Read the model definition and answer for the solid it produces. Units are mm, in the model's axes. Face numbers are marked on the shaded views. A direction names the side the tool comes from. Give positions to 0.01 mm unless a question says otherwise; leave off trailing zeros. Write each loop counter-clockwise with the first axis right and the second up, starting at its lowest first coordinate (ties: lowest second). Pieces come first, ordered by that corner, then holes.
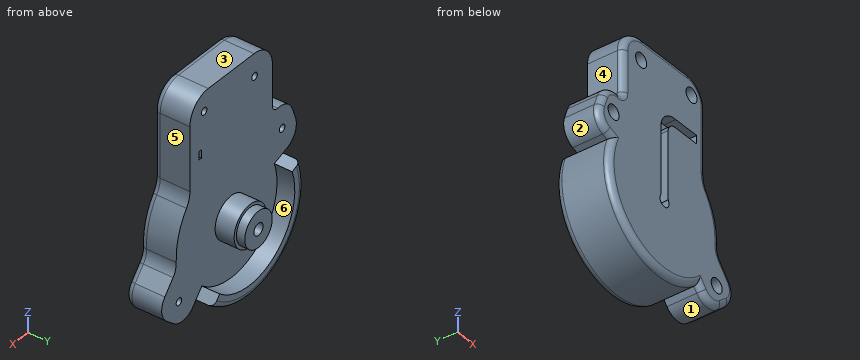
```python
from build123d import *

# Parameters (mm, degrees)
BOSS_EXTRUDE1_DEPTH = 30
SKETCH3_R           = 6
CUT_EXTRUDE2_DEPTH  = 10
CUT_EXTRUDE3_REACH  = 22
SKETCH4_R           = 3
SKETCH5_R           = 17.5
BOSS_EXTRUDE2_DEPTH = 16
SKETCH6_R           = 15
BOSS_EXTRUDE3_DEPTH = 7
BOSS_EXTRUDE4_DEPTH = 15
FILLET1_R           = 5
CUT_EXTRUDE4_REACH  = 55
SKETCH8_R           = 5
CUT_EXTRUDE5_REACH  = 32
SKETCH9_W           = 2.838035454
SKETCH9_H           = 7.000000767
CUT_EXTRUDE6_DEPTH  = 10


with BuildPart() as part:
    # Sketch1 → Boss-Extrude1 (new body)
    with BuildSketch(Plane(origin=(0, 0, 0), x_dir=(-1, 0, 0), z_dir=(0, -1, 0))):
        with BuildLine():
            Line((-155.978842812, -669.571630145), (-160.685424707, -671.259257732))
            ThreePointArc((-160.685424707, -671.259257732), (-169.1867086, -678.974834226), (-169.742287629, -690.441886175))
            Line((-169.742287629, -690.441886175), (-166.367032456, -699.855049964))
            ThreePointArc((-166.367032456, -699.855049964), (-160.015233889, -707.624119417), (-150.186716753, -709.649961495))
            ThreePointArc((-150.186716753, -709.649961495), (-146.216133795, -710.831997076), (-144.49986008, -714.602559592))
            Line((-144.49986008, -714.602559592), (-144.49986008, -749.320099104))
            ThreePointArc((-144.49986008, -749.320099104), (-138.641995704, -763.462234727), (-124.49986008, -769.320099104))
            Line((-124.49986008, -769.320099104), (-74.49986008, -769.320099104))
            ThreePointArc((-74.49986008, -769.320099104), (-60.357724456, -763.462234727), (-54.49986008, -749.320099104))
            Line((-54.49986008, -749.320099104), (-54.49986008, -695.956994369))
            ThreePointArc((-54.49986008, -695.956994369), (-53.539292845, -689.833270012), (-50.74986008, -684.297770553))
            ThreePointArc((-50.74986008, -684.297770553), (-41.916134266, -666.175796103), (-39.583621808, -646.150810326))
            ThreePointArc((-39.583621808, -646.150810326), (-38.838622962, -640.626520742), (-36.127881434, -635.755722136))
            Line((-36.127881434, -635.755722136), (-27.159022918, -624.993091916))
            ThreePointArc((-27.159022918, -624.993091916), (-23.743944015, -614.032289731), (-29.079576117, -603.867006728))
            Line((-29.079576117, -603.867006728), (-36.761788913, -597.465162731))
            ThreePointArc((-36.761788913, -597.465162731), (-47.722591099, -594.050083828), (-57.887874102, -599.38571593))
            Line((-57.887874102, -599.38571593), (-61.0887961, -603.226822328))
            ThreePointArc((-61.0887961, -603.226822328), (-133.880389498, -600.14714722), (-155.978842812, -669.571630145))
        make_face()
    extrude(amount=BOSS_EXTRUDE1_DEPTH)

    # Sketch3 → Cut-Extrude2 (cut)
    with BuildSketch(Plane.XZ.offset(30)):
        with Locations((42.52344851, 612.189403923)):
            Circle(SKETCH3_R)
        with Locations((155.092642393, 690.430908662)):
            Circle(SKETCH3_R)
        with Locations((124.976355339, 750.357765174)):
            Circle(SKETCH3_R)
        with Locations((70.026025263, 753.095100306)):
            Circle(SKETCH3_R)
    extrude(amount=-CUT_EXTRUDE2_DEPTH, mode=Mode.SUBTRACT)

    # Sketch4 → Cut-Extrude3 (cut, up to next)
    with BuildSketch(Plane.XZ.offset(20), mode=Mode.PRIVATE) as cut_extrude3_sk1:
        with Locations((42.52344851, 612.189403923)):
            Circle(SKETCH4_R)
    cut_extrude3_tool1 = extrude(cut_extrude3_sk1.sketch, amount=-CUT_EXTRUDE3_REACH, mode=Mode.PRIVATE) & part.part
    add(cut_extrude3_tool1.solids().sort_by_distance((42.523449, -20, 612.189404))[0], mode=Mode.SUBTRACT)
    # Sketch4 → Cut-Extrude3 (cut, up to next)
    with BuildSketch(Plane.XZ.offset(20), mode=Mode.PRIVATE) as cut_extrude3_sk2:
        with Locations((155.092642393, 690.430908662)):
            Circle(SKETCH4_R)
    cut_extrude3_tool2 = extrude(cut_extrude3_sk2.sketch, amount=-CUT_EXTRUDE3_REACH, mode=Mode.PRIVATE) & part.part
    add(cut_extrude3_tool2.solids().sort_by_distance((155.092642, -20, 690.430909))[0], mode=Mode.SUBTRACT)
    # Sketch4 → Cut-Extrude3 (cut, up to next)
    with BuildSketch(Plane.XZ.offset(20), mode=Mode.PRIVATE) as cut_extrude3_sk3:
        with Locations((124.976355339, 750.357765174)):
            Circle(SKETCH4_R)
    cut_extrude3_tool3 = extrude(cut_extrude3_sk3.sketch, amount=-CUT_EXTRUDE3_REACH, mode=Mode.PRIVATE) & part.part
    add(cut_extrude3_tool3.solids().sort_by_distance((124.976355, -20, 750.357765))[0], mode=Mode.SUBTRACT)
    # Sketch4 → Cut-Extrude3 (cut, up to next)
    with BuildSketch(Plane.XZ.offset(20), mode=Mode.PRIVATE) as cut_extrude3_sk4:
        with Locations((70.026025263, 753.095100306)):
            Circle(SKETCH4_R)
    cut_extrude3_tool4 = extrude(cut_extrude3_sk4.sketch, amount=-CUT_EXTRUDE3_REACH, mode=Mode.PRIVATE) & part.part
    add(cut_extrude3_tool4.solids().sort_by_distance((70.026025, -20, 753.0951))[0], mode=Mode.SUBTRACT)

    # Sketch5 → Boss-Extrude2 (add)
    with BuildSketch(Plane(origin=(0, 0, 0), x_dir=(1, 0, 0), z_dir=(0, 1, 0))):
        with Locations((99.49986008, -649.320099104)):
            Circle(SKETCH5_R)
    extrude(amount=BOSS_EXTRUDE2_DEPTH)

    # Sketch6 → Boss-Extrude3 (add)
    with BuildSketch(Plane(origin=(0, 16, 0), x_dir=(1, 0, 0), z_dir=(0, 1, 0))):
        with Locations((99.49986008, -649.320099104)):
            Circle(SKETCH6_R)
    extrude(amount=BOSS_EXTRUDE3_DEPTH)

    # Sketch7 → Boss-Extrude4 (add)
    with BuildSketch(Plane(origin=(0, 0, 0), x_dir=(1, 0, 0), z_dir=(0, 1, 0))):
        with BuildLine():
            Line((155.978842812, -669.571630145), (146.565591992, -666.196355925))
            ThreePointArc((146.565591992, -666.196355925), (128.150229883, -608.342615172), (67.490568023, -610.908994684))
            Line((67.490568023, -610.908994684), (61.0887961, -603.226822328))
            ThreePointArc((61.0887961, -603.226822328), (133.880389498, -600.14714722), (155.978842812, -669.571630145))
        make_face()
    extrude(amount=BOSS_EXTRUDE4_DEPTH)

    # Fillet1
    fillet1_edges = [part.edges().sort_by_distance(p)[0] for p in [
        (133.880389498, 15, 600.14714722),
        (23.743944015, -30, 614.032289731),
        (32.920682515, -30, 600.666084729),
        (47.722591099, -30, 594.050083828),
        (59.488335101, -30, 601.306269129),
        (133.880389498, -30, 600.14714722),
        (158.332133759, -30, 670.415443939),
        (169.1867086, -30, 678.974834226),
        (168.054660043, -30, 695.14846807),
        (160.015233889, -30, 707.624119417),
        (146.216133795, -30, 710.831997076),
        (38.838622962, -30, 640.626520742),
        (144.49986008, -30, 731.961329348),
        (138.641995704, -30, 763.462234727),
        (99.49986008, -30, 769.320099104),
        (60.357724456, -30, 763.462234727),
        (54.49986008, -30, 722.638546736),
        (53.539292845, -30, 689.833270012),
        (41.916134266, -30, 666.175796103),
        (31.643452176, -30, 630.374407026),
    ]]
    fillet(fillet1_edges, radius=FILLET1_R)


with BuildPart() as body_2:
    # Mirror1: mirrored copy
    add(part.part.mirror(Plane(origin=(0, 0, 0), x_dir=(0, 0, 1), z_dir=(1, 0, 0))))

    # Sketch8 → Cut-Extrude4 (cut, up to next)
    with BuildSketch(Plane(origin=(0, 23, 0), x_dir=(1, 0, 0), z_dir=(0, 1, 0)), mode=Mode.PRIVATE) as cut_extrude4_sk1:
        with Locations((-99.49986008, -649.320099104)):
            Circle(SKETCH8_R)
    cut_extrude4_tool1 = extrude(cut_extrude4_sk1.sketch, amount=-CUT_EXTRUDE4_REACH, mode=Mode.PRIVATE) & body_2.part
    add(cut_extrude4_tool1.solids().sort_by_distance((-99.49986, 23, 649.320099))[0], mode=Mode.SUBTRACT)

    # Sketch9 → Cut-Extrude5 (cut, up to next)
    with BuildSketch(Plane(origin=(0, 0, 0), x_dir=(1, 0, 0), z_dir=(0, 1, 0)), mode=Mode.PRIVATE) as cut_extrude5_sk1:
        with Locations((-65.749484781, -719.720058193)):
            Rectangle(SKETCH9_W, SKETCH9_H)
    cut_extrude5_tool1 = extrude(cut_extrude5_sk1.sketch, amount=-CUT_EXTRUDE5_REACH, mode=Mode.PRIVATE) & body_2.part
    add(cut_extrude5_tool1.solids().sort_by_distance((-65.749485, 0, 719.720058))[0], mode=Mode.SUBTRACT)

    # Sketch10 → Cut-Extrude6 (cut)
    with BuildSketch(Plane.XZ.offset(30)):
        with BuildLine():
            Line((-67.168502508, 716.220057809), (-87.168574927, 716.220057809))
            ThreePointArc((-87.168574927, 716.220057809), (-92.788411024, 714.505734169), (-95.54986008, 709.319612071))
            Line((-95.54986008, 709.319612071), (-95.54986008, 649.320099104))
            Line((-95.54986008, 649.320099104), (-103.44986008, 649.320099104))
            Line((-103.44986008, 649.320099104), (-103.44986008, 709.320099104))
            ThreePointArc((-103.44986008, 709.320099104), (-98.187987541, 719.642036576), (-87.168574927, 723.220058576))
            Line((-87.168574927, 723.220058576), (-67.168502508, 723.220058576))
            Line((-67.168502508, 723.220058576), (-67.168502508, 716.220057809))
        make_face()
    extrude(amount=-CUT_EXTRUDE6_DEPTH, mode=Mode.SUBTRACT)


solid = body_2.part
```
Item 1: Section B-B (y = -8.5) is taken. Write down the section's boundary in (x, z).
Result set:
outline: (-169.74, 690.44) arc R15 ccw to (-160.69, 671.26) - (-155.98, 669.57) arc R60 ccw to (-61.09, 603.23) - (-57.89, 599.39) arc R15 ccw to (-36.76, 597.47) - (-29.08, 603.87) arc R15 ccw to (-27.16, 624.99) - (-36.13, 635.76) arc R15 cw to (-39.58, 646.15) arc R60 ccw to (-50.75, 684.3) arc R20 cw to (-54.5, 695.96) - (-54.5, 749.32) arc R20 ccw to (-74.5, 769.32) - (-124.5, 769.32) arc R20 ccw to (-144.5, 749.32) - (-144.5, 714.6) arc R5 cw to (-150.19, 709.65) arc R15 ccw to (-166.37, 699.86) - close; hole circle Ø6 at (-155.09, 690.43); hole circle Ø6 at (-124.98, 750.36); hole circle Ø10 at (-99.5, 649.32); hole circle Ø6 at (-70.03, 753.1); hole (-67.17, 716.22) - (-64.33, 716.22) - (-64.33, 723.22) - (-67.17, 723.22) - close; hole circle Ø6 at (-42.52, 612.19)
Item 2: Which of the six approach directions +Z, -Z, +X, -X, +Y, -Y give full straight-line access (tool end or side, diameter ignored) to the marked faces 4, 5 and 6?
Result set:
face 4: +Z, -X, +Y, -Y
face 5: +Z, +X, +Y, -Y
face 6: +Y
Item 3: Determine the mould class of the marked faces 1, 2 and 3 for opening direction X: pulls with the +X half, pulls with the -X half, needs draft (parallel to the pull), parting line crosses it, or undercut.
Result set:
face 1: undercut
face 2: pulls with the -X half
face 3: needs draft
Item 4: Find the intervals of material crossed by line 1 along X through (y, z) = (-13, 720.5); line 2 along Z through (x, y) = (-101, 0.5); line 3 along X through (y, z) = (-27, 661), in increasing order.
Result set:
line 1: x = -144.5 to -67.17, -64.33 to -54.5
line 2: z = 589.34 to 599.34, 631.88 to 644.55, 654.09 to 666.76
line 3: x = -157.93 to -103.45, -95.55 to -41.07
Item 5: Section A-A (y = 2.5) is taken. Write down the section's boundary in (x, z), and give its area (3 significant figures).
Result set:
outline: (-155.98, 669.57) arc R60 ccw to (-61.09, 603.23) - (-67.49, 610.91) arc R50 cw to (-146.57, 666.2) - close; circle Ø35 at (-99.5, 649.32); hole circle Ø10 at (-99.5, 649.32)
area: 2,320 mm2
Item 6: Each of these flat-tipped pins is pushed along its axis until it touches: pin 1 Ø3.5 at (x, z) = (-155.09, 690.43) entering from +Y; pin 2 Ø9.5 at (x, z) = (-124.98, 750.36) entering from -Y; pin 3 Ø5 at (y, z) = (-27.5, 672.5) entering from -X; pin 4 Ø1 at (y, z) = (-13.5, 659) entering from -X. Where does it stop, or does it pass through?
Result set:
pin 1: passes through
pin 2: stops at y = -20
pin 3: stops at x = -165.92
pin 4: stops at x = -158.79
Item 7: Section C-C (y = 19) is taken. Write down the section's boundary in (x, z), and give its area (3 significant figures).
Result set:
outline: circle Ø30 at (-99.5, 649.32); hole circle Ø10 at (-99.5, 649.32)
area: 628 mm2
